Autodesk Inventor part; units mm, degrees
ref_plane "YZ Plane" through (0, 0, 0) normal (1, 0, 0) x (0, 1, 0)
ref_plane "XZ Plane" through (0, 0, 0) normal (0, 1, 0) x (-1, 0, 0)
ref_plane "XY Plane" through (0, 0, 0) normal (0, 0, 1) x (1, 0, 0)
sketch "Sketch1" plane through (0, 0, 0) normal (0, 0, 1) x (1, 0, 0)
  line L0 (-40, 15) -> (40, 15)
  line L1 (40, 15) -> (40, -15)
  line L2 (40, -15) -> (-40, -15)
  line L3 (-40, -15) -> (-40, 15)
  line L4 (-30, 7) -> (10.125, 7) construction
  line L5 (-30, 5.25) -> (10.125, 5.25)
  line L6 (10.125, 8.75) -> (-30, 8.75)
  arc A0 (-30, 8.75) -> (-30, 5.25) centre (-30, 7) ccw
  arc A1 (10.125, 5.25) -> (10.125, 8.75) centre (10.125, 7) ccw
  line L7 (-30, -7) -> (10.125, -7) construction
  line L8 (-30, -8.75) -> (10.125, -8.75)
  line L9 (10.125, -5.25) -> (-30, -5.25)
  arc A2 (-30, -5.25) -> (-30, -8.75) centre (-30, -7) ccw
  arc A3 (10.125, -8.75) -> (10.125, -5.25) centre (10.125, -7) ccw
  circle A4 centre (29, 10.5) radius 1.5
  circle A5 centre (29, -10.5) radius 1.5
  point P0 (0, 0)
  point P1 (-9.9375, 7)
  point P2 (-9.9375, -7)
  point P3 (40, 0)
  point P4 (0, -15)
  dimension "d0" = 21
  dimension "d1" = 11
  dimension "d2" = 30
  dimension "d3" = 3
  dimension "d4" = 4.5
  dimension "d5" = 80
  dimension "d6" = 3.5
  dimension "d7" = 3.5
  dimension "d8" = 10
  dimension "d10" = 10
  dimension "d11" = 8
  dimension "d12" = 8
  dimension "d13" = 18.875
  dimension "d14" = 18.875
extrude "Extrusion1" add sketch "Sketch1" along normal blind 5
sketch "Sketch2" plane through (0, 0, 5) normal (0, 0, 1) x (1, 0, 0)
  line L0 (-40, 15) -> (15, 15)
  line L1 (15, 15) -> (15, 11)
  line L2 (15, 11) -> (-40, 11)
  line L3 (-40, 11) -> (-40, 15)
  line L4 (-40, 2) -> (15, 2)
  line L5 (15, 2) -> (15, -2)
  line L6 (15, -2) -> (-40, -2)
  line L7 (-40, -2) -> (-40, 2)
  line L8 (-40, 15) -> (-40, -15)
  line L9 (-40, -15) -> (40, -15)
  line L10 (-40, -11) -> (15, -11)
  line L11 (15, -11) -> (15, -15)
  line L12 (15, -15) -> (-40, -15)
  line L13 (-40, -15) -> (-40, -11)
  point P0 (0, 0)
  point P1 (15, 0)
  dimension "d17" = 4
  dimension "d18" = 4
  dimension "d19" = 4
  dimension "d20" = 55
extrude "Extrusion2" add sketch "Sketch2" along normal blind 1
chamfer "Chamfer1" distance 2 angle 45 8 edges at (-9.9375, 5.25, 0) (11.875, 7, 0) (-9.9375, 8.75, 0) (-31.75, 7, 0) (-9.9375, -8.75, 0) (11.875, -7, 0) (-9.9375, -5.25, 0) (-31.75, -7, 0)
equation "\"d10\" = d8"
equation "\"d14\" = d13"
equation "\"d18\" = d17"
equation "\"d19\" = d17"
Input: part model. Units: mm. Frame: model coordinates. A direction names the side the tool comes from. Give positions to 0.01 mm unless a question says otherwise; leave off trailing zeros. Loops run counter-clockwise (first coordinate to the right, second up) from the corner with the lowest first, then second, coordinate; pieces in that order, holes last. Notation, with made-up numbers: (40.25, 70) - (63.25, 70) arc R22 ccw to (63.25, 100) - close; hole circle Ø4 at (30, -37.5). An arc over 180 degrees is marked (long way). Use CSV: the item, a comma, the result in double quotes. Start each with the question number.
Item 1: Section C-C on z = 1.05. Return loops of the section in (x, y) (3 decimals), then the cut area to 3 significant figures.
Item 2: Line query: line 1 (Y direction, x = -5, z = 5.7); line 2 (Y direction, x = 29, z = 3.35); line 3 (X direction, y = 4.75, z = 1.05). Output: solid intervals per line, ascending.
Item 3: Contact query for flat-ended pins moving along their axis: P1, Ø0.8, axis at y = 14, z = 5.5, coming from the +X side; P2, Ø2.5, axis at x = 29, y = 10.5, coming from the +Z side. Output: stop coordinate, or through.
Item 4: Section D-D on x = 29. Return loops of the section in (y, z), then the cut area to 3 significant figures.
Item 5: Section B-B on x = -9. Return loops of the section in (y, z), then the cut area to 3 significant figures.
Item 6: Mould query, pull axis X, two halves, no side actions, for faces 4 (the flat face through (8, 4, 5)), 5 (the cylindrical face through (27.5, 10.43, 2.46)), 6 (the cylindrical face through (11.875, 7.038, 3.479)), 7 (the flat face through (-40, 0, 3)). Classes: pulls with the +X half, pulls with the -X half, needs draft (parallel to the pull), parting line crosses it, or undercut.
Item 7: Section A-A on y = -7. Return loops of the section in (x, z) (3 decimals).
Item 8: Reachability of faces 1 (the cylindrical face through (-31.75, -7.04, 3.48)), 2 (the conical face through (-32.32, 6.95, 1.43)), 3 (the flat face through (-13, 13, 6)) from +Z, -Z, +X, -X, +Y, -Y: full face, straight path, thin tool, end or side. Return the list, or none.
Ans:
1,outline,"(-40, -15) - (40, -15) - (40, 15) - (-40, 15) - close; hole (-30, -9.7) - (10.125, -9.7) arc R2.7 ccw to (10.125, -4.3) - (-30, -4.3) arc R2.7 ccw to start; hole (-30, 4.3) - (10.125, 4.3) arc R2.7 ccw to (10.125, 9.7) - (-30, 9.7) arc R2.7 ccw to start; hole circle Ø3 at (29, -10.5); hole circle Ø3 at (29, 10.5)"
1,area,"1,910 mm2"
2,line 1,"y = -15 to -11, -2 to 2, 11 to 15"
2,line 2,"y = -15 to -12, -9 to 9, 12 to 15"
2,line 3,"x = -40 to -31.49, 11.62 to 40"
3,P1,"stops at x = 15"
3,P2,"passes through"
4,outline,"(-15, 0) - (-12, 0) - (-12, 5) - (-15, 5) - close; (-9, 0) - (9, 0) - (9, 5) - (-9, 5) - close; (12, 0) - (15, 0) - (15, 5) - (12, 5) - close"
4,area,"120 mm2"
5,outline,"(-15, 0) - (-10.75, 0) - (-8.75, 2) - (-8.75, 5) - (-11, 5) - (-11, 6) - (-15, 6) - close; (-5.25, 2) - (-3.25, 0) - (3.25, 0) - (5.25, 2) - (5.25, 5) - (2, 5) - (2, 6) - (-2, 6) - (-2, 5) - (-5.25, 5) - close; (8.75, 2) - (10.75, 0) - (15, 0) - (15, 6) - (11, 6) - (11, 5) - (8.75, 5) - close"
5,area,"119 mm2"
6,face 4,"needs draft"
6,face 5,"undercut"
6,face 6,"undercut"
6,face 7,"pulls with the -X half"
7,outline,"(-40, 0) - (-33.75, 0) - (-31.75, 2) - (-31.75, 5) - (-40, 5) - close; (11.875, 2) - (13.875, 0) - (40, 0) - (40, 5) - (11.875, 5) - close"
8,face 1,"+Z, -Z"
8,face 2,"-Z"
8,face 3,"+Z, +X, -X, +Y, -Y"
